Autodesk Inventor part; units mm, degrees
ref_plane "YZ Plane" through (0, 0, 0) normal (1, 0, 0) x (0, 1, 0)
ref_plane "XZ Plane" through (0, 0, 0) normal (0, 1, 0) x (-1, 0, 0)
ref_plane "XY Plane" through (0, 0, 0) normal (0, 0, 1) x (1, 0, 0)
sketch "Sketch1" plane through (0, 0, 0) normal (0, 0, 1) x (1, 0, 0)
  line L0 (0, 0) -> (80, 0)
  line L1 (80, 0) -> (80, 36)
  line L2 (80, 36) -> (0, 36)
  line L3 (0, 36) -> (0, 0)
  circle A0 centre (27.5, 30.464) radius 1.7
  circle A1 centre (27.5, 5.064) radius 1.7
  circle A2 centre (76, 30.464) radius 1.7
  circle A3 centre (76, 5.064) radius 1.7
  circle A4 centre (4, 31.365) radius 1.7
  circle A5 centre (19.558, 31.365) radius 1.7
  dimension "d0" = 36
  dimension "d1" = 80
  dimension "d2" = 3.4
  dimension "d3" = 3.4
  dimension "d4" = 3.4
  dimension "d5" = 3.4
  dimension "d6" = 3.4
  dimension "d7" = 3.4
  dimension "d8" = 5.536
  dimension "d10" = 5.536
  dimension "d11" = 48.5
  dimension "d12" = 25.4
  dimension "d13" = 48.5
  dimension "d14" = 25.4
  dimension "d16" = 15.558
  dimension "d17" = 4.635
  dimension "d18" = 4.635
  dimension "d39" = 4
  dimension "d40" = 4
  dimension "d41" = 4
extrude "Extrusion1" add sketch "Sketch1" along normal blind 3.5
sketch "Sketch2" plane through (0, 0, 3.5) normal (0, 0, 1) x (1, 0, 0)
  line L0 (30, 34) -> (60, 34)
  line L1 (60, 34) -> (60, 36)
  line L2 (60, 36) -> (30, 36)
  line L3 (30, 36) -> (30, 34)
  line L4 (80, 36) -> (0, 36)
  line L5 (0, 36) -> (0, 0)
  line L6 (80, 0) -> (80, 36)
  dimension "d22" = 2
  dimension "d24" = 30
  dimension "d42" = 20
extrude "Extrusion2" add sketch "Sketch2" along normal blind 5.1
sketch "Sketch3" plane through (30, 34, 3.5) normal (0, -1, 0) x (1, 0, 0)
  line L0 (0, 3.1) -> (30, 3.1)
  line L1 (30, 3.1) -> (30, 5.1)
  line L2 (30, 5.1) -> (0, 5.1)
  line L3 (0, 5.1) -> (0, 3.1)
  line L4 (0, 5.1) -> (30, 5.1)
  line L5 (0, 0) -> (0, 5.1)
  line L6 (30, 0) -> (30, 5.1)
  line L7 (-30, 0) -> (50, 0)
  point P0 (-30, -3.5)
  dimension "d27" = 3.1
extrude "Extrusion3" add sketch "Sketch3" along normal blind 11.75 contours L3 L2 L1 L0
chamfer "Chamfer1" distance 5 angle 45 2 edges at (30, 22.25, 7.6) (60, 22.25, 7.6)
chamfer "Chamfer2" distance 2 angle 45 6 edges at (25.8, 30.464, 3.5) (25.8, 5.064, 3.5) (74.3, 5.064, 3.5) (74.3, 30.464, 3.5) (2.3, 31.365, 3.5) (17.858, 31.365, 3.5)
chamfer "Chamfer3" distance 1 angle 45 2 edges at (0, 0, 1.75) (80, 0, 1.75)
properties part number "PowerMountingBracket"
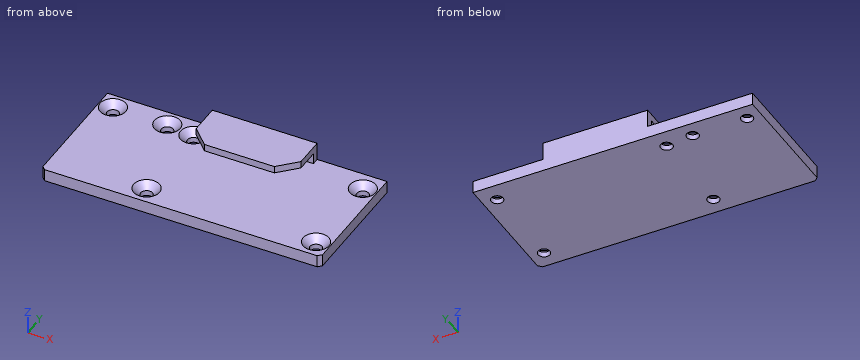
Work out the finished part from the listing and answer in its coordinate system (mm). Give positions to 0.01 mm unless a question says otherwise; leave off trailing zeros. Order: outer loops, then holes, each group sorted by start corner. A loop starts at its lowest first (then second) coordinate and runs counter-clockwise, first axis right, second up.
1. Section D-D, the plane x = 46 is taken. Determine the outline of the cut face in (y, z).
Result sheet:
outline: (0, 0) - (36, 0) - (36, 8.6) - (22.25, 8.6) - (22.25, 6.6) - (34, 6.6) - (34, 3.5) - (0, 3.5) - close
2. Section A-A, the plane x = 76 is taken. Determine the outline of the cut face in (y, z).
Result sheet:
outline: (0, 0) - (3.36, 0) - (3.36, 1.5) - (1.36, 3.5) - (0, 3.5) - close; (6.76, 0) - (28.76, 0) - (28.76, 1.5) - (26.76, 3.5) - (8.76, 3.5) - (6.76, 1.5) - close; (32.16, 0) - (36, 0) - (36, 3.5) - (34.16, 3.5) - (32.16, 1.5) - close
3. Section C-C, the plane z = 7.75 is taken. Determine the outline of the cut face in (x, y), and give its area (4 significant figures).
Result sheet:
outline: (30, 27.25) - (35, 22.25) - (55, 22.25) - (60, 27.25) - (60, 36) - (30, 36) - close
area: 387.5 mm2
4. Section B-B, the plane x = 4 is taken. Determine the outline of the cut face in (y, z) (3 decimals), and give its area (3 significant figures).
Result sheet:
outline: (0, 0) - (29.665, 0) - (29.665, 1.5) - (27.665, 3.5) - (0, 3.5) - close; (33.065, 0) - (36, 0) - (36, 3.5) - (35.065, 3.5) - (33.065, 1.5) - close
area: 110 mm2
5. Each of these flat-tipped pins is pushed along its axis until it touches: P1, Ø1.5, axis at x = 42.5, z = 6, coming from the -Y side; P2, Ø5.5, axis at x = 76, y = 30.464, coming from the -Z side; P3, Ø2, axis at x = 27.5, y = 30.464, coming from the -Z side; P4, Ø1.5, axis at y = 31.5, z = 6, coming from the +X side. Where does it stop, or does it pass through?
Result sheet:
P1: stops at y = 22.25
P2: stops at z = 0
P3: passes through
P4: stops at x = 60
6. Straight lines are drawn through the part: L1, parallel to Y at x = 27.5, z = 0.7; L2, parallel to Y at x = 4, z = 0.7 (3 decimals); L3, parallel to X at y = 29, z = 3. For each, find the intervals that lie inside material, in ascending order.
Result sheet:
L1: y = 0 to 3.36, 6.76 to 28.76, 32.16 to 36
L2: y = 0 to 29.665, 33.065 to 36
L3: x = 0 to 1.84, 6.16 to 17.4, 21.71 to 24.65, 30.35 to 73.15, 78.85 to 80
